from build123d import *

# Parameters (mm, degrees)
F0_W        = 100
F0_H        = 100
F1_DEPTH    = 100
F2_W        = 88.9338813722
F2_H        = 88.2601328194
F3_DEPTH    = 90
F5_DEPTH    = 185
F6_T        = 5
F6_T3_DEPTH = 100
F6_T5_DEPTH = 98.2601328194
F6_T7_DEPTH = 98.9338813722
F7_W        = 90
F7_H        = 95
F8_DEPTH    = 8
F10_DEPTH   = 25
F11_R       = 23.6849070482
F11_R_2     = 18.1970048193
F12_DEPTH   = 25
F13_W       = 74.0287862718
F13_H       = 40.3192453086
F14_DEPTH   = 9
F15_W       = 33.1602711231
F15_H       = 63.8056004047
F16_DEPTH   = 25
F17_W       = 95
F17_H       = 277
F18_DEPTH   = 31
F19_W       = 29.5484475791
F19_H       = 21.4659199119
F20_DEPTH   = 25


# Not quite as in the source:
# - a shell that OpenCascade refuses in one call is made with other operations: the cavity is built on its own and cut out


with BuildPart() as f1:
    # F0 (on Front) → F1 (new body)
    with BuildSketch(Plane.XZ):
        with Locations((-6.5152887255, 3.7536189136)):
            Rectangle(F0_W, F0_H)
    extrude(amount=F1_DEPTH)

    # F2 (on face) → F3 (cut)
    with BuildSketch(Plane.XZ.offset(100)):
        with Locations((-6.6661592573, 4.4211242348)):
            Rectangle(F2_W, F2_H)
    extrude(amount=-F3_DEPTH, mode=Mode.SUBTRACT)

    # F4 (on face) → F5 (join)
    with BuildSketch(Plane.XY.offset(53.7536189136)):
        Polygon((-56.5152887255, -100), (43.4847112745, -100), (43.4847112745, -33.4126986563), (43.4847112745, 0), (-56.5152887255, 0), align=None)
    extrude(amount=F5_DEPTH)

    # F6: shell of thickness 5, made by hand


with BuildPart() as f6_core1:
    # F6_t2: copy of F1
    add(f1.part)

    # the walls: a layer under each face that stays
    f6_faces = [f6_core1.faces().sort_by_distance(p)[0] for p in [
        (43.4847112745, -50, 96.2536189136),
        (-6.5152887255, 0, 96.2536189136),
        (-56.5152887255, -50, 96.2536189136),
        (-51.1330999434, -55, 4.4211242348),
        (-6.6661592573, -10, 4.4211242348),
        (-6.6661592573, -55, -39.7089421749),
        (37.8007814288, -55, 4.4211242348),
        (-6.6661592573, -55, 48.5511906445),
        (-6.5152887255, -50, -46.2463810864),
    ]]
    thicken(f6_faces, amount=-F6_T, mode=Mode.SUBTRACT)

    # F6_s4 → F6_t3 (cut)
    with BuildSketch(Plane.XZ.offset(5)):
        Polygon((-51.0830999434, 48.5011906445), (-56.1330999434, 48.5511906445), (-56.1330999434, 53.5511906445), (-51.1330999434, 53.5511906445), align=None)
        Polygon((-51.0830999434, -39.6589421749), (-56.1330999434, -39.7089421749), (-56.1330999434, -44.7089421749), (-51.1330999434, -44.7089421749), align=None)
        Polygon((37.7507814288, -39.6589421749), (37.8007814288, -44.7089421749), (42.8007814288, -44.7089421749), (42.8007814288, -39.7089421749), align=None)
        Polygon((37.7507814288, 48.5011906445), (42.8007814288, 48.5511906445), (42.8007814288, 53.5511906445), (37.8007814288, 53.5511906445), align=None)
    extrude(amount=F6_T3_DEPTH, mode=Mode.SUBTRACT)

    # F6_s6 → F6_t5 (cut)
    with BuildSketch(Plane.XY.offset(-44.7089421749)):
        Polygon((-51.0830999434, -10.05), (-56.1330999434, -10), (-56.1330999434, -5), (-51.1330999434, -5), align=None)
        Polygon((37.7507814288, -10.05), (37.8007814288, -5), (42.8007814288, -5), (42.8007814288, -10), align=None)
    extrude(amount=F6_T5_DEPTH, mode=Mode.SUBTRACT)

    # F6_s8 → F6_t7 (cut)
    with BuildSketch(Plane.YZ.offset(-56.1330999434)):
        Polygon((-10.05, 48.5011906445), (-5, 48.5511906445), (-5, 53.5511906445), (-10, 53.5511906445), align=None)
        Polygon((-10.05, -39.6589421749), (-5, -39.7089421749), (-5, -44.7089421749), (-10, -44.7089421749), align=None)
    extrude(amount=F6_T7_DEPTH, mode=Mode.SUBTRACT)


with BuildPart() as f1_1:
    add(f1.part)

    # what is left inside the walls is the cavity
    f6_cavity = [f6_core1.part.solids().sort_by_distance(p)[0] for p in [
        (38.434711, -68.333333, 146.152405),
    ]]
    add(f6_cavity, mode=Mode.SUBTRACT)

    # F7 (on face) → F8 (join)
    with BuildSketch(Plane.XY.offset(238.7536189136)):
        with Locations((-6.5152887255, -52.5)):
            Rectangle(F7_W, F7_H)
    extrude(amount=-F8_DEPTH)

    # F9 (on face) → F10 (join)
    with BuildSketch(Plane(origin=(-56.5152887255, 0, 0), x_dir=(0, -1, 0), z_dir=(-1, 0, 0))):
        with BuildLine():
            ThreePointArc((0, 189.510354193), (12.2569085004, 194.5873319266), (17.333886234, 206.844240427))
            ThreePointArc((17.333886234, 206.844240427), (12.2569085004, 219.1011489274), (0, 224.178126661))
            Line((0, 224.178126661), (0, 189.510354193))
        make_face()
        with BuildLine():
            Line((0, 189.510354193), (0, 224.178126661))
            ThreePointArc((0, 224.178126661), (-17.333886234, 206.844240427), (0, 189.510354193))
        make_face()
        with BuildLine():
            Line((0, -23.6541135693), (0, 23.6541135693))
            ThreePointArc((0, 23.6541135693), (-15.7209434523, 0), (0, -23.6541135693))
        make_face()
    extrude(amount=-F10_DEPTH)

    # F11 (on face) → F12 (join)
    with BuildSketch(Plane.YZ.offset(43.4847112745)):
        with Locations((-11.2718828022, 0)):
            Circle(F11_R)
        with Locations((0, 216.0427719355)):
            Circle(F11_R_2)
    extrude(amount=-F12_DEPTH)

    # F13 (on face) → F14 (cut)
    with BuildSketch(Plane(origin=(0, 0, -46.2463810864), x_dir=(1, 0, 0), z_dir=(0, 0, -1))):
        with Locations((-6.1139781028, 59.594200924)):
            Rectangle(F13_W, F13_H)
    extrude(amount=-F14_DEPTH, mode=Mode.SUBTRACT)

    # F15 (on face) → F16 (cut)
    with BuildSketch(Plane(origin=(0, 0, 48.5511906445), x_dir=(1, 0, 0), z_dir=(0, 0, -1))):
        with Locations((9.9139763042, 41.9028002024)):
            Rectangle(F15_W, F15_H)
    extrude(amount=-F16_DEPTH, mode=Mode.SUBTRACT)

    # F17 (on face) → F18 (join)
    with BuildSketch(Plane.XZ.offset(100)):
        with Locations((-9.0152887255, 92.2536189136)):
            Rectangle(F17_W, F17_H)
    extrude(amount=-F18_DEPTH)

    # F19 (on face) → F20 (cut)
    with BuildSketch(Plane.YZ.offset(43.4847112745)):
        with Locations((-26.0461065918, -10.7329599559)):
            Rectangle(F19_W, F19_H)
    extrude(amount=-F20_DEPTH, mode=Mode.SUBTRACT)


solid = f1_1.part
Design review of the part built by this model. Coordinates are the model's own, in mm. A direction names the side the tool comes from. Round coordinates to 2 decimals unless told otherwise and drop trailing zeros. Write each loop counter-clockwise with the first axis right and the second up, starting at its lowest first coordinate (ties: lowest second). Pieces come first, ordered by that corner, then holes. Notation, with made-up numbers: M 36,10.25 L 73,10.25 A37 ccw 73,48.25 Z; hole C 45,14.5 d5. An arc over 180 degrees is marked long. One line per item, written item: value. Start each with the question number.
1. Take a section at D-D on y = -44. State the section outline as (x, z) points.
2. Draft analysis for pull direction X (two halves, no side actions). For faces 1 (the face through (18.485, -20, 11)), 2 (the face through (-56.515, -41, 94)), 3 (the face through (31.16, 12.41, -0.36)), state which applies: pulls with the +X half, pulls with the -X half, needs draft (parallel to the pull), parting line crosses it, or undercut.
3. For faces 4 (the face through (31, -23, 0)), 5 (the face through (-31.515, 6, 0)), 6 (the face through (-44.19, 15.717, 0.421)), 7 (the face through (28.28, -15.85, -23.24)), list the 3-axis set-ups (+Z, -Z, +X, -X, +Y, -Y) from which the entire face can be reached by the end or side of a thin tool; tool diameter is ignored.
4. Take a section at C-C on x = 13.5. State the section outline as (y, z) points, then the cut area to 3 significant figures.
5. Take a section at A-A on z = 77.5. State the section outline as (x, y) points, then the cut area to 3 significant figures.
6. Clearance check with flat-ended pins moving along their axes: P1, Ø5, axis at x = -11.5, y = -58.5, coming from the -Z side; P2, Ø6, axis at x = 23.5, z = 181.5, coming from the +Y side. State where each tip first meets the part, or that it passes through.
7. Take a section at B-B on x = -17.5. State the section outline as (y, z) points.
8. To check wall thickness, follow probe 1 along Y at (x, z) = (-20.5, 5); probe 2 along Y at (x, z) = (-47.5, 97.5); probe 3 along X at (y, z) = (-66, 151). State the ranges of each line that lie inside material, in increasing order. Write a range as from..to.
Computed:
1. outline: M -56.52,-46.25 L -43.13,-46.25 L -43.13,-39.71 L -51.13,-39.71 L -51.13,48.55 L -6.67,48.55 L -6.67,53.55 L -51.52,53.55 L -51.52,230.75 L 38.48,230.75 L 38.48,53.55 L 26.49,53.55 L 26.49,48.55 L 37.8,48.55 L 37.8,-39.71 L 30.9,-39.71 L 30.9,-46.25 L 43.48,-46.25 L 43.48,238.75 L -56.52,238.75 Z
2. face 1: undercut
2. face 2: pulls with the -X half
2. face 3: needs draft
3. face 4: +X
3. face 5: +Z, -Z, +Y
3. face 6: +X, -X, +Y
3. face 7: none
4. outline: M -100,-46.25 L -69,-46.25 L -69,230.75 L -5,230.75 L -5,53.55 L -10,53.55 L -10,-39.71 L -39.43,-39.71 L -39.43,-46.25 L 0,-46.25 L 0,238.75 L -100,238.75 Z
4. area: 11,500 mm²
5. outline: M -56.52,-100 L 43.48,-100 L 43.48,0 L -56.52,0 Z; hole M -51.52,-69 L 38.48,-69 L 38.48,-5 L -51.52,-5 Z
5. area: 4,240 mm²
6. P1: stops at z = 48.55
6. P2: stops at y = 0
7. outline: M -100,-46.25 L -69,-46.25 L -69,48.55 L -10,48.55 L -10,-39.71 L -39.43,-39.71 L -39.43,-46.25 L 0,-46.25 L 0,238.75 L -100,238.75 Z; hole M -69,53.55 L -5,53.55 L -5,230.75 L -69,230.75 Z
8. probe 1: y = -100..-69, -10..0
8. probe 2: y = -100..-69, -5..0
8. probe 3: x = -56.52..-51.52, 38.48..43.48
